```python
from build123d import *

# Parameters (mm, degrees)
SKETCH_1_R      = 25
EXTRUDE_1_DEPTH = 3
HOLE_WIZARD_1_D = 3.5
HOLE_WIZARD_2_D = 18
HOLE_WIZARD_3_D = 3


with BuildPart() as part:
    # 草图1 → 凸台-拉伸1 (new body)
    with BuildSketch(Plane(origin=(0, 0, 0), x_dir=(1, 0, 0), z_dir=(0, 1, 0))):
        with Locations(Location((0, 0, 0), (0, 0, 270))):
            Circle(SKETCH_1_R)
    extrude(amount=EXTRUDE_1_DEPTH)

    # 孔1 (through all)
    with Locations(Plane(origin=(0, 3, 0), x_dir=(1, 0, 0), z_dir=(0, 1, 0))):
        with Locations((0, 20), (-17.320508076, -10), (17.320508076, -10)):
            Hole(HOLE_WIZARD_1_D / 2)

    # 孔2 (through all)
    with Locations(Plane(origin=(0, 3, 0), x_dir=(1, 0, 0), z_dir=(0, 1, 0))):
        with Locations((0, 0)):
            Hole(HOLE_WIZARD_2_D / 2)

    # 孔3 (through all)
    with Locations(Plane(origin=(0, 3, 0), x_dir=(1, 0, 0), z_dir=(0, 1, 0))):
        with Locations((-10.825317547, 6.25), (0, -12.5), (10.825317547, 6.25)):
            Hole(HOLE_WIZARD_3_D / 2)


solid = part.part
```
The model under review builds one solid part; all positions refer to its coordinate system, in mm. Round coordinates to 2 decimals unless told otherwise and drop trailing zeros. Write each loop counter-clockwise with the first axis right and the second up, starting at its lowest first coordinate (ties: lowest second). Pieces come first, ordered by that corner, then holes. Notation, with made-up numbers: M 17,-3 L 32,-3 A21 cw 32,15 Z; hole C -37,41 d4. An arc over 180 degrees is marked long. Use CSV: the item, a comma, the result in double quotes. Start each with the question number.
(1) We need section D-D, the plane x = -7. State the section outline as (y, z) points.
(2) We need section A-A, the plane y = 1.15. State the section outline as (x, z) points.
(3) Clearance check with flat-ended pins moving along their axes: P1, Ø1.8, axis at x = -10.83, z = -6.25, coming from the -Y side; P2, Ø1.5, axis at x = 17, y = 1.5, coming from the +Z side; P3, Ø1, axis at x = 10.5, z = 15.5, coming from the -Y side; P4, Ø1, axis at y = 2.5, z = -8.5, coming from the +X side. State where each tip first meets the part, or that it passes through.
(4) We need section C-C, the plane z = -2. State the section outline as (x, y) points.
(5) The part is to be moulded in two halves that separate along Z. For faces 1 (the face through (18.61, 1.479, 8.817)), 2 (the face through (7.509, 1.479, 23.846)), 3 (the face through (-18.99, 1.48, 9.47)), 4 (the face through (-11, 0, 0)), say which applies: +Z half, -Z half, draft (parallel to the pull), parting line (faces both ways), or undercut.
(6) For line 1 along X through (y, z) = (2.15, 10); line 2 along Z through (x, y) = (6, 0.9); line 3 along Z through (x, y) = (-4.5, 0.7), list the stretches that pass through material, from the lowest coordinate up.
(7) We need section B-B, the plane x = 0. State the section outline as (y, z) points.
Findings:
1,outline,"M 0,-24 L 3,-24 L 3,-5.66 L 0,-5.66 Z; M 0,5.66 L 3,5.66 L 3,24 L 0,24 Z"
2,outline,"C 0,0 d50; hole C -17.32,10 d3.5; hole C -10.83,-6.25 d3; hole C 0,0 d18; hole C 0,-20 d3.5; hole C 0,12.5 d3; hole C 10.83,-6.25 d3; hole C 17.32,10 d3.5"
3,P1,"through"
3,P2,"z = 19"
3,P3,"y = 0"
3,P4,"x = 23.69"
4,outline,"M -24.92,0 L -8.77,0 L -8.77,3 L -24.92,3 Z; M 8.77,0 L 24.92,0 L 24.92,3 L 8.77,3 Z"
5,face 1,"undercut"
5,face 2,"parting line"
5,face 3,"undercut"
5,face 4,"draft"
6,line 1,"-22.91 to -19.07, -15.57 to 15.57, 19.07 to 22.91"
6,line 2,"-24.27 to -6.71, 6.71 to 24.27"
6,line 3,"-24.59 to -7.79, 7.79 to 24.59"
7,outline,"M 0,-25 L 3,-25 L 3,-21.75 L 0,-21.75 Z; M 0,-18.25 L 3,-18.25 L 3,-9 L 0,-9 Z; M 0,9 L 3,9 L 3,11 L 0,11 Z; M 0,14 L 3,14 L 3,25 L 0,25 Z"
